Autodesk Inventor part; units mm, degrees
ref_plane "YZ Plane" through (0, 0, 0) normal (1, 0, 0) x (0, 1, 0)
ref_plane "XZ Plane" through (0, 0, 0) normal (0, 1, 0) x (-1, 0, 0)
ref_plane "XY Plane" through (0, 0, 0) normal (0, 0, 1) x (1, 0, 0)
sketch "Sketch1" plane through (0, 0, 0) normal (0, 1, 0) x (-1, 0, 0)
  line L0 (-4.445, 19.939) -> (4.445, 19.939)
  line L1 (4.445, 19.939) -> (4.445, -19.939)
  line L2 (4.445, -19.939) -> (-4.445, -19.939)
  line L3 (-4.445, -19.939) -> (-4.445, 19.939)
  line L4 (-4.445, 19.939) -> (4.445, -19.939) construction
  line L5 (4.445, 19.939) -> (-4.445, -19.939) construction
  circle A0 centre (0, 0) radius 2
  dimension "d0" = 8.89
  dimension "d1" = 39.878
  dimension "d2" = 4
extrude "Extrusion1" add sketch "Sketch1" along normal blind 5.08
properties part number "BeltMount"
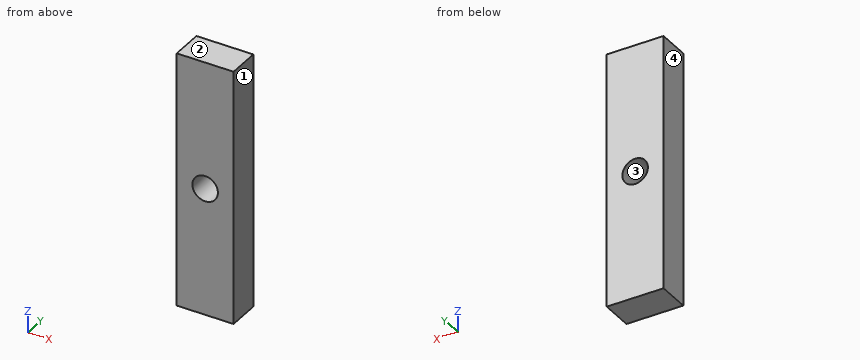
Read the model definition and answer for the solid it produces. Units are mm, in the model's axes. Face numbers are marked on the shaded views. Round coordinates to 2 decimals unless told otherwise and drop trailing zeros. Loops run counter-clockwise (first coordinate to the right, second up) from the corner with the lowest first, then second, coordinate; pieces in that order, holes last.
Q1. Determine the mould class of the marked faces 1, 2, 3 and 4 for opening direction X: released by +X, released by -X, zero draft, split by the parting line, or undercut.
Q2. Section B-B on x = 0 is taken. Write down the section's boundary in (y, z), and give its area (3 significant figures).
Q3. Section C-C on y = 3 is taken. Write down the section's boundary in (x, z) (3 decimals), and give its area (3 significant figures).
Q4. Section A-A on z = 0 is taken. Write down the section's boundary in (x, y) (3 decimals).
Q5. Consider probe 1 along Z at (x, y) = (0, 2.7); probe 2 along Z at (x, y) = (-1.25, 4). Determine where each line is inside the solid, lowest interval first.
Output:
1. face 1: released by +X
1. face 2: zero draft
1. face 3: undercut
1. face 4: released by -X
2. outline: (0, -19.94) - (5.08, -19.94) - (5.08, -2) - (0, -2) - close; (0, 2) - (5.08, 2) - (5.08, 19.94) - (0, 19.94) - close
2. area: 182 mm2
3. outline: (-4.445, -19.939) - (4.445, -19.939) - (4.445, 19.939) - (-4.445, 19.939) - close; hole circle Ø4 at (0, 0)
3. area: 342 mm2
4. outline: (-4.445, 0) - (-2, 0) - (-2, 5.08) - (-4.445, 5.08) - close; (2, 0) - (4.445, 0) - (4.445, 5.08) - (2, 5.08) - close
5. probe 1: z = -19.94 to -2, 2 to 19.94
5. probe 2: z = -19.94 to -1.56, 1.56 to 19.94
